from build123d import *

# Parameters (mm, degrees)
SKETCH1_R           = 3.5
BOSS_EXTRUDE1_DEPTH = 5
CUT_EXTRUDE1_DEPTH  = 5
FILLET1_R           = 0.25


with BuildPart() as part:
    # Sketch1 → Boss-Extrude1 (new body)
    with BuildSketch(Plane(origin=(0, 0, 0), x_dir=(1, 0, 0), z_dir=(0, 1, 0))):
        with Locations(Location((0, 0, 0), (0, 0, 270))):
            Circle(SKETCH1_R)
    extrude(amount=BOSS_EXTRUDE1_DEPTH)

    # Sketch2 → Cut-Extrude1 (cut)
    with BuildSketch(Plane(origin=(0, 5, 0), x_dir=(1, 0, 0), z_dir=(0, 1, 0))):
        with BuildLine():
            Line((1.4, -1.949358869), (1.4, 1.949358869))
            ThreePointArc((1.4, 1.949358869), (0, 2.4), (-1.4, 1.949358869))
            Line((-1.4, 1.949358869), (-1.4, -1.949358869))
            ThreePointArc((-1.4, -1.949358869), (0, -2.4), (1.4, -1.949358869))
        make_face()
    extrude(amount=-CUT_EXTRUDE1_DEPTH, mode=Mode.SUBTRACT)

    # Fillet1
    fillet1_edges = [part.edges().sort_by_distance(p)[0] for p in [
        (1.4, 2.5, 1.949358869),
        (-1.4, 2.5, 1.949358869),
        (-1.4, 2.5, -1.949358869),
        (1.4, 2.5, -1.949358869),
    ]]
    fillet(fillet1_edges, radius=FILLET1_R)


solid = part.part
Source: CAD feature listing. Evaluate the final solid. Frame: model axes, mm. A direction names the side the tool comes from. Coordinates: 2 decimals unless noted, no trailing zeros. Order: outer loops, then holes, each group sorted by start corner. A loop starts at its lowest first (then second) coordinate and runs counter-clockwise, first axis right, second up. Notation, with made-up numbers: M 21,-9 L 70,-9 A16 ccw 70,15 Z; hole C -15.75,69.5 d1. An arc over 180 degrees is marked long. Write each question's results on one line, items separated by ' | '. Start each with the question number.
Item 1: Cut plane C-C (z = 0). Return loops of the section in (x, y), and give its area (3 significant figures).
Item 2: Cut plane B-B (y = 1.75). Return loops of the section in (x, z), and give its area (3 significant figures).
Item 3: Cut plane A-A (x = 0). Return loops of the section in (y, z), and give its area (3 significant figures).
Item 4: First-contact query: pin 1 Ø1 at (x, y) = (-1, 3) entering from -Z. Flat tip, straight axial feed; report the tip coordinate or a pass-through.
Item 5: Draft query along X for faces 1 (the face through (-2, 0, 0)), 2 (the face through (-3.417, 2.465, -0.759)), 3 (the face through (0, 2.5, -2.4)), 4 (the face through (1.4, 3, 0)). Return one class per face: pulls with the +X half, pulls with the -X half, needs draft (parallel to the pull), parting line crosses it, or undercut.
Item 6: Line query: probe 1 along X at (y, z) = (3.35, 0); probe 2 along X at (y, z) = (0.45, -0.75); probe 3 along Z at (x, y) = (0.75, 1.3). Output: solid intervals per line, ascending.
Item 7: Cut plane D-D (z = 3). Return loops of the section in (x, y).
Item 8: Set-up query: faces 5 (the face through (0, 2.5, 2.4)), 6 (the face through (-2, 5, 0)). Return all of +Z, -Z, +X, -X, +Y, -Y with unobstructed straight access to the full face (end or side cutting, diameter ignored); none if empty.
Checked values:
1) outline: M -3.5,0 L -1.4,0 L -1.4,5 L -3.5,5 Z; M 1.4,0 L 3.5,0 L 3.5,5 L 1.4,5 Z | area: 21.0 mm2
2) outline: C 0,0 d7; hole M -1.4,-1.82 A0.25 ccw -1.28,-2.03 A2.4 ccw 1.28,-2.03 A0.25 ccw 1.4,-1.82 L 1.4,1.82 A0.25 ccw 1.28,2.03 A2.4 ccw -1.28,2.03 A0.25 ccw -1.4,1.82 Z | area: 25.9 mm2
3) outline: M 0,-3.5 L 5,-3.5 L 5,-2.4 L 0,-2.4 Z; M 0,2.4 L 5,2.4 L 5,3.5 L 0,3.5 Z | area: 11.0 mm2
4) pin 1: stops at z = -3.46
5) face 1: needs draft | face 2: parting line crosses it | face 3: undercut | face 4: undercut
6) probe 1: x = -3.5 to -1.4, 1.4 to 3.5 | probe 2: x = -3.42 to -1.4, 1.4 to 3.42 | probe 3: z = -3.42 to -2.28, 2.28 to 3.42
7) outline: M -1.8,0 L 1.8,0 L 1.8,5 L -1.8,5 Z
8) face 5: +Y, -Y | face 6: +Z, -Z, +X, -X, +Y
